from build123d import *

# Parameters (mm, degrees)
EXTRUDE_1_DEPTH     = 15
SKETCH_6_R          = 3.5
CUT_EXTRUDE_2_DEPTH = 15
EXTRUDE_START       = 17
SKETCH_11_R         = 15
SKETCH_11_R_2       = 3.5
EXTRUDE_3_DEPTH     = 17
SKETCH_12_R         = 10.1
CUT_EXTRUDE_6_DEPTH = 2
SKETCH_13_R         = 0.5
CUT_EXTRUDE_7_DEPTH = 3


with BuildPart() as part:
    # ｽｹｯﾁ1 → ﾎﾞｽ - 押し出し1 (new body)
    with BuildSketch(Plane.XY):
        with BuildLine():
            Line((10.546944731, 68.165925034), (9.641814145, 68.990666647))
            ThreePointArc((9.641814145, 68.990666647), (-9.131421435, 69.400300104), (-13.594616806, 51.160726074))
            Line((-13.594616806, 51.160726074), (4.986432096, 11.313538113))
            ThreePointArc((4.986432096, 11.313538113), (5.221931994, 9.524738795), (4.388829079, 7.924362985))
            Line((4.388829079, 7.924362985), (-40.303464689, -36.767930783))
            ThreePointArc((-40.303464689, -36.767930783), (-41.182112782, -38.903012739), (-40.283913759, -41.029943849))
            ThreePointArc((-40.283913759, -41.029943849), (41.397896806, -39.905690573), (39.524106652, 41.762363359))
            Line((39.524106652, 41.762363359), (37.916838192, 43.226882625))
            Line((37.916838192, 43.226882625), (10.546944731, 68.165925034))
        make_face()
        with BuildLine():
            ThreePointArc((5.093338956, 1.55780505), (7.735603832, 2.390907965), (9.933582661, 0.704339492))
            Line((9.933582661, 0.704339492), (27.046217634, -35.993824637))
            ThreePointArc((27.046217634, -35.993824637), (27.212084573, -38.085077821), (25.967336583, -39.773702754))
            ThreePointArc((25.967336583, -39.773702754), (-1.972837213, -47.459012983), (-29.17877254, -37.481318454))
            ThreePointArc((-29.17877254, -37.481318454), (-30.330146685, -35.299826939), (-29.457223039, -32.992756945))
            Line((-29.457223039, -32.992756945), (5.093338956, 1.55780505))
        make_face(mode=Mode.SUBTRACT)
        with BuildLine():
            ThreePointArc((35.231836325, -31.858557864), (32.560090836, -32.813013733), (30.287744354, -31.114293205))
            Line((30.287744354, -31.114293205), (-2.054746852, 38.244403012))
            ThreePointArc((-2.054746852, 38.244403012), (-1.895310582, 41.077194163), (0.553480425, 42.510214831))
            ThreePointArc((0.553480425, 42.510214831), (5.039223996, 43.371793408), (9.057681155, 45.543478261))
            ThreePointArc((9.057681155, 45.543478261), (10.270904088, 46.091905397), (11.601973614, 46.061309233))
            ThreePointArc((11.601973614, 46.061309233), (45.455779175, 13.784851815), (35.231836325, -31.858557864))
        make_face(mode=Mode.SUBTRACT)
    extrude(amount=EXTRUDE_1_DEPTH)

    # ｽｹｯﾁ6 → ｶｯﾄ - 押し出し2 (cut)
    with BuildSketch(Plane.XY.offset(15)):
        with Locations((0, 57.5)):
            Circle(SKETCH_6_R)
    extrude(amount=-CUT_EXTRUDE_2_DEPTH, mode=Mode.SUBTRACT)

    # ｽｹｯﾁ11 → ﾎﾞｽ - 押し出し3 (add)
    with BuildSketch(Plane(origin=(0, 0, 0), x_dir=(-1, 0, 0), z_dir=(0, 0, -1)).offset(EXTRUDE_START)):
        with Locations((0, 57.5)):
            Circle(SKETCH_11_R)
        with Locations(Location((0, 57.5, 0), (0, 0, 180))):
            Circle(SKETCH_11_R_2, mode=Mode.SUBTRACT)
    extrude(amount=-EXTRUDE_3_DEPTH)

    # ｽｹｯﾁ12 → ｶｯﾄ - 押し出し6 (cut)
    with BuildSketch(Plane(origin=(0, 0, -17), x_dir=(-1, 0, 0), z_dir=(0, 0, -1))):
        with Locations((0, 57.5)):
            Circle(SKETCH_12_R)
    extrude(amount=-CUT_EXTRUDE_6_DEPTH, mode=Mode.SUBTRACT)

    # ｽｹｯﾁ13 → ｶｯﾄ - 押し出し7 (cut)
    with BuildSketch(Plane(origin=(0, 0, -15), x_dir=(-1, 0, 0), z_dir=(0, 0, -1))):
        with Locations((-3.5, 65.5)):
            Circle(SKETCH_13_R)
        with Locations((0, 65.5)):
            Circle(SKETCH_13_R)
        with Locations((3.5, 65.5)):
            Circle(SKETCH_13_R)
        with Locations((8, 57.5)):
            Circle(SKETCH_13_R)
        with Locations((8, 61)):
            Circle(SKETCH_13_R)
        with Locations((8, 54)):
            Circle(SKETCH_13_R)
        with Locations((0, 49.5)):
            Circle(SKETCH_13_R)
        with Locations((3.5, 49.5)):
            Circle(SKETCH_13_R)
        with Locations((-3.5, 49.5)):
            Circle(SKETCH_13_R)
        with Locations((-8, 57.5)):
            Circle(SKETCH_13_R)
        with Locations((-8, 54)):
            Circle(SKETCH_13_R)
        with Locations((-8, 61)):
            Circle(SKETCH_13_R)
    extrude(amount=-CUT_EXTRUDE_7_DEPTH, mode=Mode.SUBTRACT)


solid = part.part
Input: part model. Units: mm. Frame: model coordinates. A direction names the side the tool comes from. Coordinates: 2 decimals unless noted, no trailing zeros. Loops run counter-clockwise (first coordinate to the right, second up) from the corner with the lowest first, then second, coordinate; pieces in that order, holes last. Notation, with made-up numbers: (84.5, -11.75) -> (93.5, -11.75) arc R36 ccw to (93.5, 27.25) -> close; hole circle Ø2 at (64, -19.75). An arc over 180 degrees is marked (long way). One line per item, written item: value.
(1) Cut plane B-B (y = -25). Output: boundary loops of the cut face in (x, z).
Answer below:
outline: (-28.54, 0) -> (-21.46, 0) -> (-21.46, 15) -> (-28.54, 15) -> close; (21.92, 0) -> (27.44, 0) -> (27.44, 15) -> (21.92, 15) -> close; (40.39, 0) -> (51.78, 0) -> (51.78, 15) -> (40.39, 15) -> close
(2) Cut plane D-D (z = -2). Output: boundary loops of the cut face in (x, y).
Answer below:
outline: circle Ø30 at (0, 57.5); hole circle Ø7 at (0, 57.5)
(3) Cut plane C-C (x = 41). Output: boundary loops of the cut face in (y, z).
Answer below:
outline: (-40.31, 0) -> (-23.98, 0) -> (-23.98, 15) -> (-40.31, 15) -> close; (23.98, 0) -> (40.31, 0) -> (40.31, 15) -> (23.98, 15) -> close
(4) Set-up query: faces 1 (the face through (-4, 58, -15)), 2 (the face through (-30.328, -35.335, 7.395)), 3 (the face through (-4.434, 31.516, 7.395)). Return all of +Z, -Z, +X, -X, +Y, -Y with unobstructed straight access to the full face (end or side cutting, diameter ignored); none if empty.
Answer below:
face 1: -Z
face 2: +Z, -Z
face 3: +Z, -Z, -X
(5) Pin query (flat end, axial travel): pin 1 Ø1.5 at (y, z) = (1, 1.5) entering from -X; pin 2 Ø11 at (x, y) = (0, 57.5) entering from -Z; pin 3 Ø4 at (x, y) = (14, -13.5) entering from -Z; pin 4 Ø0.5 at (x, y) = (8, 57.5) entering from -Z. Return the tip coordinate at first contact, or that it passes through.
Answer below:
pin 1: stops at x = -3.29
pin 2: stops at z = -15
pin 3: passes through
pin 4: stops at z = -12
(6) Ray query, line 1 along Y through (x, z) = (0, -13); line 2 along X through (y, z) = (65.5, -13.7); line 3 along Y through (x, z) = (8, -13.65). Return the intervals inside material, ascending.
Answer below:
line 1: y = 42.5 to 49, 50 to 54, 61 to 65, 66 to 72.5
line 2: x = -12.69 to -4, -3 to -0.5, 0.5 to 3, 4 to 12.69
line 3: y = 44.81 to 53.5, 54.5 to 57, 58 to 60.5, 61.5 to 70.19
(7) Draft query along X for faces 4 (the face through (-17.644, -14.109, 7.395)), 5 (the face through (-5.43, 66.016, -16.014)), 6 (the face through (12, 3, 15)). Return one class per face: pulls with the +X half, pulls with the -X half, needs draft (parallel to the pull), parting line crosses it, or undercut.
Answer below:
face 4: pulls with the -X half
face 5: undercut
face 6: needs draft
